Job drawing, mm, ordinate dimensions from the low corner. One solid piece. Give positions to 0.01 mm unless a question says otherwise; leave off trailing zeros. Loops run counter-clockwise (first coordinate to the right, second up) from the corner with the lowest first, then second, coordinate; pieces in that order, holes last. Notation, with made-up numbers: (80, -35) - (89, -35) arc R12 ccw to (89, -27) - close; hole circle Ø2 at (4.5, 28). An arc over 180 degrees is marked (long way). Use a Markdown table: item, result.
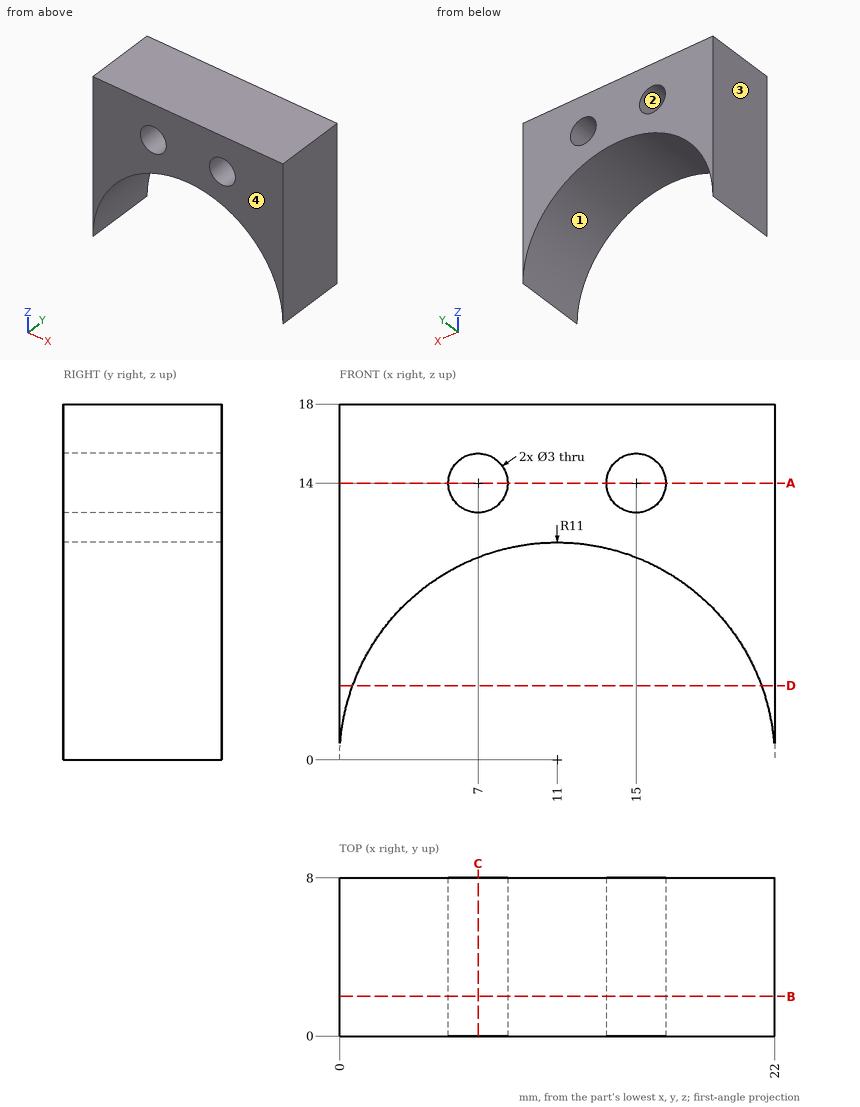
(1) Slice it at A-A, the plane z = 14. Write the cut outline in (x, y).
Computed:
| item | result |
|---|---|
| outline | (0, 0) - (5.5, 0) - (5.5, 8) - (0, 8) - close; (8.5, 0) - (13.5, 0) - (13.5, 8) - (8.5, 8) - close; (16.5, 0) - (22, 0) - (22, 8) - (16.5, 8) - close |
(2) Pin check, flat tip, straight feed: P1, Ø6, axis at x = 16, z = 7, coming from the -Y side. Stop position of the tip, or through.
Computed:
| item | result |
|---|---|
| P1 | y = 0 |
(3) Slice it at D-D, the plane z = 3.75. Write the cut outline in (x, y).
Computed:
| item | result |
|---|---|
| outline | (0, 0) - (0.66, 0) - (0.66, 8) - (0, 8) - close; (21.34, 0) - (22, 0) - (22, 8) - (21.34, 8) - close |
(4) Mould opens along X. For the marked faces 1, 2, 3 and 4 say: pulls with the +X half, pulls with the -X half, needs draft (parallel to the pull), parting line crosses it, or undercut.
Computed:
| item | result |
|---|---|
| face 1 | undercut |
| face 2 | undercut |
| face 3 | pulls with the -X half |
| face 4 | needs draft |
(5) Drill centre lines: probe 1 along X at (y, z) = (5.75, 14.75); probe 2 along X at (y, z) = (1, 15.25); probe 3 along X at (y, z) = (5.75, 9). Where is each one in solid material? Low to high. Write a range as [from, to].
Computed:
| item | result |
|---|---|
| probe 1 | [0, 5.7], [8.3, 13.7], [16.3, 22] |
| probe 2 | [0, 6.17], [7.83, 14.17], [15.83, 22] |
| probe 3 | [0, 4.68], [17.32, 22] |
(6) Slice it at B-B, the plane y = 2. Write the cut outline in (x, z), plus the area to 3 significant figures.
Computed:
| item | result |
|---|---|
| outline | (0, 0) arc R11 cw to (22, 0) - (22, 18) - (0, 18) - close; hole circle Ø3 at (7, 14); hole circle Ø3 at (15, 14) |
| area | 192 mm² |
(7) Slice it at C-C, the plane x = 7. Write the cut outline in (y, z), plus the area to 3 significant figures.
Computed:
| item | result |
|---|---|
| outline | (0, 10.25) - (8, 10.25) - (8, 12.5) - (0, 12.5) - close; (0, 15.5) - (8, 15.5) - (8, 18) - (0, 18) - close |
| area | 38.0 mm² |
